```python
from build123d import *

# Parameters (mm, degrees)
BOSS_EXTRUDE4_DEPTH                                 = 2
BOSS_EXTRUDE5_START                                 = 2
BOSS_EXTRUDE5_DEPTH                                 = 2
BOSS_EXTRUDE6_DEPTH                                 = 2
FILLET1_R                                           = 2
CBORE_FOR_3_BINDING_HEAD_MACHINE_SCREW1_D           = 2.794
CBORE_FOR_3_BINDING_HEAD_MACHINE_SCREW1_CBORE_D     = 5.95376
CBORE_FOR_3_BINDING_HEAD_MACHINE_SCREW1_CBORE_DEPTH = 1.4986
SKETCH10_R                                          = 1.5
CUT_EXTRUDE1_DEPTH                                  = 5
SKETCH9_R                                           = 1.5
CUT_EXTRUDE2_DEPTH                                  = 5


with BuildPart() as part:
    # Sketch1 → Boss-Extrude4 (new body)
    with BuildSketch(Plane.XY):
        with BuildLine():
            Line((37.090015594, -18.299625702), (38, -0.099937578))
            Line((38, -0.099937578), (38, 33.052037892))
            Line((38, 33.052037892), (33.662977857, 75.458476622))
            ThreePointArc((33.662977857, 75.458476622), (31.715138161, 79.301265628), (27.694112953, 80.84802453))
            Line((27.694112953, 80.84802453), (6.305887047, 80.84802453))
            ThreePointArc((6.305887047, 80.84802453), (2.284861839, 79.301265628), (0.337022143, 75.458476622))
            Line((0.337022143, 75.458476622), (-4, 33.052037892))
            Line((-4, 33.052037892), (-4, -0.099937578))
            Line((-4, -0.099937578), (-3.090015594, -18.299625702))
            ThreePointArc((-3.090015594, -18.299625702), (-1.232851956, -22.347283877), (2.902498439, -24))
            Line((2.902498439, -24), (31.097501561, -24))
            ThreePointArc((31.097501561, -24), (35.232851956, -22.347283877), (37.090015594, -18.299625702))
        make_face()
    extrude(amount=BOSS_EXTRUDE4_DEPTH)

    # Sketch5 → Boss-Extrude5 (add)
    with BuildSketch(Plane(origin=(0, 0, 0), x_dir=(-1, 0, 0), z_dir=(0, 0, -1)).offset(BOSS_EXTRUDE5_START)):
        with BuildLine():
            Line((-33.662977857, 75.458476622), (-38, 33.052037892))
            Line((-38, 33.052037892), (-38, -0.099937578))
            Line((-38, -0.099937578), (-37.090015594, -18.299625702))
            ThreePointArc((-37.090015594, -18.299625702), (-35.232851956, -22.347283877), (-31.097501561, -24))
            Line((-31.097501561, -24), (-2.902498439, -24))
            ThreePointArc((-2.902498439, -24), (1.232851956, -22.347283877), (3.090015594, -18.299625702))
            Line((3.090015594, -18.299625702), (4, -0.099937578))
            Line((4, -0.099937578), (4, 33.052037892))
            Line((4, 33.052037892), (-0.337022143, 75.458476622))
            ThreePointArc((-0.337022143, 75.458476622), (-2.284861839, 79.301265628), (-6.305887047, 80.84802453))
            Line((-6.305887047, 80.84802453), (-27.694112953, 80.84802453))
            ThreePointArc((-27.694112953, 80.84802453), (-31.715138161, 79.301265628), (-33.662977857, 75.458476622))
        make_face()
        with BuildLine():
            Line((-31.097501561, -22), (-2.902498439, -22))
            ThreePointArc((-2.902498439, -22), (-0.145598176, -20.898189251), (1.092510916, -18.199750468))
            Line((1.092510916, -18.199750468), (2, -0.049968789))
            Line((2, -0.049968789), (2, 32.950031211))
            Line((2, 32.950031211), (-2.326643778, 75.254992592))
            ThreePointArc((-2.326643778, 75.254992592), (-3.625203575, 77.816851929), (-6.305887047, 78.84802453))
            Line((-6.305887047, 78.84802453), (-27.694112953, 78.84802453))
            ThreePointArc((-27.694112953, 78.84802453), (-30.374796425, 77.816851929), (-31.673356222, 75.254992592))
            Line((-31.673356222, 75.254992592), (-36, 32.950031211))
            Line((-36, 32.950031211), (-36, -0.049968789))
            Line((-36, -0.049968789), (-35.092510916, -18.199750468))
            ThreePointArc((-35.092510916, -18.199750468), (-33.854401824, -20.898189251), (-31.097501561, -22))
        make_face(mode=Mode.SUBTRACT)
    extrude(amount=-BOSS_EXTRUDE5_DEPTH)

    # Sketch6 → Boss-Extrude6 (add)
    with BuildSketch(Plane(origin=(0, 0, 0), x_dir=(-1, 0, 0), z_dir=(0, 0, -1))):
        with BuildLine():
            Line((-30.625, 65.84802453), (-3.375, 65.84802453))
            Line((-3.375, 65.84802453), (0, 32.84802453))
            Line((0, 32.84802453), (0, 0))
            Line((0, 0), (-0.904993762, -18.099875234))
            ThreePointArc((-0.904993762, -18.099875234), (-1.524048308, -19.449094626), (-2.902498439, -20))
            Line((-2.902498439, -20), (-31.097501561, -20))
            ThreePointArc((-31.097501561, -20), (-32.475951692, -19.449094626), (-33.095006238, -18.099875234))
            Line((-33.095006238, -18.099875234), (-34, 0))
            Line((-34, 0), (-34, 32.84802453))
            Line((-34, 32.84802453), (-30.625, 65.84802453))
        make_face()
    extrude(amount=BOSS_EXTRUDE6_DEPTH)

    # Fillet1
    fillet1_edges = [part.edges().sort_by_distance(p)[0] for p in [
        (30.625, 65.84802453, -1),
        (3.375, 65.84802453, -1),
    ]]
    fillet(fillet1_edges, radius=FILLET1_R)

    # CBORE for #3 Binding Head Machine Screw1 (through all)
    with Locations(Plane.XY.offset(2)):
        with Locations((24.663824929, 71.84802453), (9.664488304, 71.84802453)):
            CounterBoreHole(CBORE_FOR_3_BINDING_HEAD_MACHINE_SCREW1_D / 2, CBORE_FOR_3_BINDING_HEAD_MACHINE_SCREW1_CBORE_D / 2, CBORE_FOR_3_BINDING_HEAD_MACHINE_SCREW1_CBORE_DEPTH)

    # Sketch10 → Cut-Extrude1 (cut)
    with BuildSketch(Plane.XY.offset(2)):
        with Locations((17, 6.476050157)):
            Circle(SKETCH10_R)
    extrude(amount=-CUT_EXTRUDE1_DEPTH, mode=Mode.SUBTRACT)

    # Sketch9 → Cut-Extrude2 (cut)
    with BuildSketch(Plane.XY.offset(2)):
        with Locations((17, 6.476050157)):
            Circle(SKETCH9_R)
        with Locations((17, 26.476050157)):
            Circle(SKETCH9_R)
    extrude(amount=-CUT_EXTRUDE2_DEPTH, mode=Mode.SUBTRACT)


solid = part.part
```
Verification items for the finished model (mm, model axes). A direction names the side the tool comes from. Round coordinates to 2 decimals unless told otherwise and drop trailing zeros. Write each loop counter-clockwise with the first axis right and the second up, starting at its lowest first coordinate (ties: lowest second). Pieces come first, ordered by that corner, then holes.
1. Section check A-A on x = 17. Enter the section's corners in (y, z).
2. Scan lines: L1, parallel to Y at x = 17, z = -1.2; L2, parallel to Y at x = 17, z = 0.6; L3, parallel to Y at x = 12.5, z = -1.4. Record each from-to range of solid material in increasing order.
3. Section check B-B on z = -0.95. State how many separate pieces and enclosed holes the cut face has, plus the area to 3 significant figures.
4. Access from +Z, -Z, +X, -X, +Y, -Y to the whole of each face (thin tool, end or side, straight path). Record for faces 4 (the cylindrical face through (31.67, 79.34, -0.03)), 5 (the flat face through (0.133, 53.806, -1.014)), 6 (the flat face through (26, 71, 0.501)).
5. Draft check along Y on faces 1 (the flat face through (38, 17, 0)), 2 (the cylindrical face through (35.28, -22.3, -0.03)), 3 (the flat face through (34, 16, -1)). Enter one of: +Y half, -Y half, draft (parallel to the pull), parting line (faces both ways), or undercut.
6. Gauge pin test, flat ends, axial feed: P1, Ø2.5, axis at x = 17, y = 26.48, coming from the -Z side; P2, Ø1.8, axis at x = 8, y = 70.5, coming from the +Z side; P3, Ø5.5, axis at x = 9.66, y = 71.85, coming from the -Z side; P4, Ø5, axis at x = 24.66, y = 71.85, coming from the +Z side. Record the tip position at first contact, or that the pin passes through.
Answer:
1. outline: (-24, -2) - (-22, -2) - (-22, 0) - (-20, 0) - (-20, -2) - (4.98, -2) - (4.98, 2) - (-24, 2) - close; (7.98, -2) - (24.98, -2) - (24.98, 2) - (7.98, 2) - close; (27.98, -2) - (65.85, -2) - (65.85, 0) - (78.85, 0) - (78.85, -2) - (80.85, -2) - (80.85, 2) - (27.98, 2) - close
2. L1: y = -24 to -22, -20 to 4.98, 7.98 to 24.98, 27.98 to 65.85, 78.85 to 80.85
2. L2: y = -24 to 4.98, 7.98 to 24.98, 27.98 to 80.85
2. L3: y = -24 to -22, -20 to 65.85, 78.85 to 80.85
3. separate pieces: 2
3. enclosed holes: 3
3. area: 3,300 mm2
4. face 4: +Z, -Z, +X, +Y
4. face 5: -Z
4. face 6: +Z
5. face 1: draft
5. face 2: -Y half
5. face 3: undercut
6. P1: passes through
6. P2: stops at z = 2
6. P3: stops at z = 0
6. P4: stops at z = 0.5
